CAD build for the part. Positions are in the model's coordinates, mm. A direction names the side the tool comes from. Coordinates: 2 decimals unless noted, no trailing zeros. Order: outer loops, then holes, each group sorted by start corner. A loop starts at its lowest first (then second) coordinate and runs counter-clockwise, first axis right, second up. Notation, with made-up numbers: (-2.5, 38) - (29.5, 38) arc R30 ccw to (29.5, 65) - close; hole circle Ø4 at (-38.5, -9). An arc over 180 degrees is marked (long way). Return JSON: item names as keys, results as strings.
from build123d import *

# Parameters (mm, degrees)
F0_R     = 33
F0_R_2   = 14
F1_DEPTH = 5
F2_R     = 25.5
F2_R_2   = 14
F3_DEPTH = 3
F4_R     = 20
F4_R_2   = 14
F5_DEPTH = 4


with BuildPart() as f1:
    # F0 (on Front) → F1 (new body)
    with BuildSketch(Plane.XZ):
        Circle(F0_R)
        Circle(F0_R_2, mode=Mode.SUBTRACT)
    extrude(amount=F1_DEPTH)

    # F2 (on face) → F3 (cut)
    with BuildSketch(Plane.XZ.offset(5)):
        Circle(F2_R)
        Circle(F2_R_2, mode=Mode.SUBTRACT)
    extrude(amount=-F3_DEPTH, mode=Mode.SUBTRACT)

    # F4 (on face) → F5 (join)
    with BuildSketch(Plane.XZ.offset(2)):
        Circle(F4_R)
        Circle(F4_R_2, mode=Mode.SUBTRACT)
    extrude(amount=F5_DEPTH)

    # F6 (on Top) → F7 (revolve, cut)
    with BuildSketch(Plane.XY):
        with BuildLine():
            ThreePointArc((20.3859657049, -2), (17.2039851896, -9.6819805153), (24.8859657049, -6.5))
            ThreePointArc((24.8859657049, -6.5), (23.5679462203, -3.3180194847), (20.3859657049, -2))
        make_face()
    revolve(axis=Axis((0, -6, 0), (0, -1, 0)), mode=Mode.SUBTRACT)


solid = f1.part
Item 1: Wall check: L1, parallel to Z at x = 0, y = -3.55; L2, parallel to Z at x = 9, y = -4.2; L3, parallel to Y at x = 8, z = 18.5. Give the ranges that are in metal, low to high. Write a range as [from, to].
Findings below:
{"L1": "z = [-33, -25.5], [-16.99, -14], [14, 16.99], [25.5, 33]", "L2": "z = [-31.75, -23.86], [-13.85, -10.72], [10.72, 13.85], [23.86, 31.75]", "L3": "y = [-2, 0]"}
Item 2: Band-saw the part on D-D, the plane z = 23.5. List the corners of the cut face in (x, y), then the cut area to 3 significant figures.
Findings below:
{"outline": "(-23.17, -5) - (-9.9, -5) - (-9.9, -2) - (9.9, -2) - (9.9, -5) - (23.17, -5) - (23.17, 0) - (-23.17, 0) - close", "area": "172 mm²"}
Item 3: Band-saw the part on C-C, the plane y = -3.8. List the corners of the cut face in (x, z).
Findings below:
{"outline": "circle Ø66 at (0, 0); circle Ø33.57 at (0, 0); hole circle Ø51 at (0, 0); hole circle Ø28 at (0, 0)"}
Item 4: Drop flat-ended pins along their axis: P1, Ø2, axis at y = -3.5, z = -20, coming from the +X side; P2, Ø2, axis at y = -5, z = 26, coming from the -X side; P3, Ø6, axis at x = 10, z = -20.5, coming from the -Y side. Give the stop position or say it passes through.
Findings below:
{"P1": "stops at x = 26.98", "P2": "stops at x = -21.54", "P3": "stops at y = -5"}
Item 5: Mould opens along Z. For faces 1 (the cylindrical face through (30.5, -2.5, -12.6)), 2 (the cylindrical face through (12.932, -2.958, -5.362)), 3 (the flat face through (9, -6, -11)) say: released by +Z, released by -Z, zero draft, split by the parting line, or undercut.
Findings below:
{"face 1": "split by the parting line", "face 2": "undercut", "face 3": "zero draft"}
Item 6: Which spindle directions (+Z, -Z, +X, -X, +Y, -Y) get a long thin tool onto all of the face, cutting with end or side? Do faces 4 (the flat face through (-0.5, 0, -14.2)), 5 (the flat face through (17, -5, -19.4)). Say none if no direction does.
Findings below:
{"face 4": "+Z, -Z, +X, -X, +Y", "face 5": "-Y"}
